Here's how the part is built. I have some questions about the finished solid (model axes, mm). Round coordinates to 2 decimals unless told otherwise and drop trailing zeros. Order: outer loops, then holes, each group sorted by start corner. A loop starts at its lowest first (then second) coordinate and runs counter-clockwise, first axis right, second up. Notation, with made-up numbers: M 66,-27 L 118,-27 A20 cw 118,8 Z; hole C 10,11.25 d1. An arc over 180 degrees is marked long. Write item = value, one per line. Start each with the question number.
Item 1: I'm going to push flat-ended pins straight in: P1, Ø2, axis at y = 3.5, z = 77, coming from the +X side; P2, Ø1.5, axis at y = 3, z = 86.5, coming from the +X side; P3, Ø1.5, axis at y = -0.5, z = 17, coming from the -X side. Where does each tip first touch, or does it pass through?
Item 2: Please list where these lines run through material, in increasing order: L1, parallel to Y at x = 0.25, z = 55.5; L2, parallel to Y at x = -1.25, z = 46.5; L3, parallel to X at y = 0, z = 21.5.
Item 3: I want a section at A-A, the plane z = 13.5. List the corners of the cut face in (x, y) for me.
Item 4: I want a section at B-B, the plane y = -3. List the corners of the cut face in (x, z) for me.
Item 5: We'd pull the mould along X, two halves only. Please class faces 1 (the face through (3.73, -2.2, 44.37)), 2 (the face through (0.035, 3.195, 93.959)), 3 (the face through (-3.77, -2.13, 44.37)), 4 (the face through (-1.5, 0.07, 50.7)): pulls with the +X half, pulls with the -X half, needs draft (parallel to the pull), parting line crosses it, or undercut.
```python
from build123d import *
from OCP.BRepFilletAPI import BRepFilletAPI_MakeChamfer

# Parameters (mm, degrees)
VYSUNOUT1_DEPTH          = 100
ZKOSIT2_SIZE             = 10
ZKOSIT2_SIZE2            = 2.867453858
SKICA2_R                 = 1.5
ODEBRAT_VYSUNUT_M1_DEPTH = 101.218511264


with BuildPart() as part:
    # Skica1 → Vysunout1 (new body)
    with BuildSketch(Plane.XY):
        Polygon((2.5, -4.330127019), (5, 0), (2.5, 4.330127019), (-2.5, 4.330127019), (-5, 0), (-2.5, -4.330127019), align=None)
    extrude(amount=VYSUNOUT1_DEPTH)

    # Zkosit2: one chamfer whose edges measure the first distance from different faces: ONE call of the kernel's chamfer builder (chamfer() names one face for all edges)
    zkosit2_edges_1 = [part.edges().sort_by_distance(p)[0] for p in [
        (3.75, 2.165063509, 100),
    ]]
    zkosit2_side_1 = [part.faces().sort_by_distance(p)[0] for p in [
        (3.75, 2.165063509, 50),
    ]]
    zkosit2_edges_2 = [part.edges().sort_by_distance(p)[0] for p in [
        (0, 4.330127019, 100),
    ]]
    zkosit2_side_2 = [part.faces().sort_by_distance(p)[0] for p in [
        (0, 4.330127019, 50),
    ]]
    zkosit2_edges_3 = [part.edges().sort_by_distance(p)[0] for p in [
        (-3.75, 2.165063509, 100),
    ]]
    zkosit2_side_3 = [part.faces().sort_by_distance(p)[0] for p in [
        (-3.75, 2.165063509, 50),
    ]]
    zkosit2_edges_4 = [part.edges().sort_by_distance(p)[0] for p in [
        (-3.75, -2.165063509, 100),
    ]]
    zkosit2_side_4 = [part.faces().sort_by_distance(p)[0] for p in [
        (-3.75, -2.165063509, 50),
    ]]
    zkosit2_edges_5 = [part.edges().sort_by_distance(p)[0] for p in [
        (0, -4.330127019, 100),
    ]]
    zkosit2_side_5 = [part.faces().sort_by_distance(p)[0] for p in [
        (0, -4.330127019, 50),
    ]]
    zkosit2_edges_6 = [part.edges().sort_by_distance(p)[0] for p in [
        (3.75, -2.165063509, 100),
    ]]
    zkosit2_side_6 = [part.faces().sort_by_distance(p)[0] for p in [
        (3.75, -2.165063509, 50),
    ]]
    zkosit2 = BRepFilletAPI_MakeChamfer(part.part.solid().wrapped)
    for e in zkosit2_edges_1:
        zkosit2.Add(ZKOSIT2_SIZE, ZKOSIT2_SIZE2, e.wrapped, zkosit2_side_1[0].wrapped)  # the first distance lies on this face
    for e in zkosit2_edges_2:
        zkosit2.Add(ZKOSIT2_SIZE, ZKOSIT2_SIZE2, e.wrapped, zkosit2_side_2[0].wrapped)  # the first distance lies on this face
    for e in zkosit2_edges_3:
        zkosit2.Add(ZKOSIT2_SIZE, ZKOSIT2_SIZE2, e.wrapped, zkosit2_side_3[0].wrapped)  # the first distance lies on this face
    for e in zkosit2_edges_4:
        zkosit2.Add(ZKOSIT2_SIZE, ZKOSIT2_SIZE2, e.wrapped, zkosit2_side_4[0].wrapped)  # the first distance lies on this face
    for e in zkosit2_edges_5:
        zkosit2.Add(ZKOSIT2_SIZE, ZKOSIT2_SIZE2, e.wrapped, zkosit2_side_5[0].wrapped)  # the first distance lies on this face
    for e in zkosit2_edges_6:
        zkosit2.Add(ZKOSIT2_SIZE, ZKOSIT2_SIZE2, e.wrapped, zkosit2_side_6[0].wrapped)  # the first distance lies on this face
    add(Compound.cast(zkosit2.Shape()), mode=Mode.REPLACE)

    # Skica2 → Odebrat vysunutím1 (cut, through all)
    with BuildSketch(Plane.XY.offset(100)):
        Circle(SKICA2_R)
    extrude(amount=-ODEBRAT_VYSUNUT_M1_DEPTH, mode=Mode.SUBTRACT)


solid = part.part
```
Filled in:
q1.P1 = 3.56
q1.P2 = 3.7
q1.P3 = -5
q2.L1 = -4.33 to -1.48, 1.48 to 4.33
q2.L2 = -4.33 to -0.83, 0.83 to 4.33
q2.L3 = -5 to -1.5, 1.5 to 5
q3.outline = M -5,0 L -2.5,-4.33 L 2.5,-4.33 L 5,0 L 2.5,4.33 L -2.5,4.33 Z; hole C 0,0 d3
q4.outline = M -3.27,0 L 3.27,0 L 3.27,90 L 1.73,94.64 L -1.73,94.64 L -3.27,90 Z
q5.face_1 = pulls with the +X half
q5.face_2 = needs draft
q5.face_3 = pulls with the -X half
q5.face_4 = undercut
